Drawing for the job (mm, zero at the part's lowest x, y, z). A direction names the side the tool comes from. Round coordinates to 2 decimals unless told otherwise and drop trailing zeros. Write each loop counter-clockwise with the first axis right and the second up, starting at its lowest first coordinate (ties: lowest second). Pieces come first, ordered by that corner, then holes. Notation, with made-up numbers: (-34.5, 55.25) - (-2.5, 55.25) arc R29 ccw to (-2.5, 82.25) - close; hole circle Ø4 at (13.25, 15.5). An arc over 180 degrees is marked (long way). One line per question, with ' | ' between items.
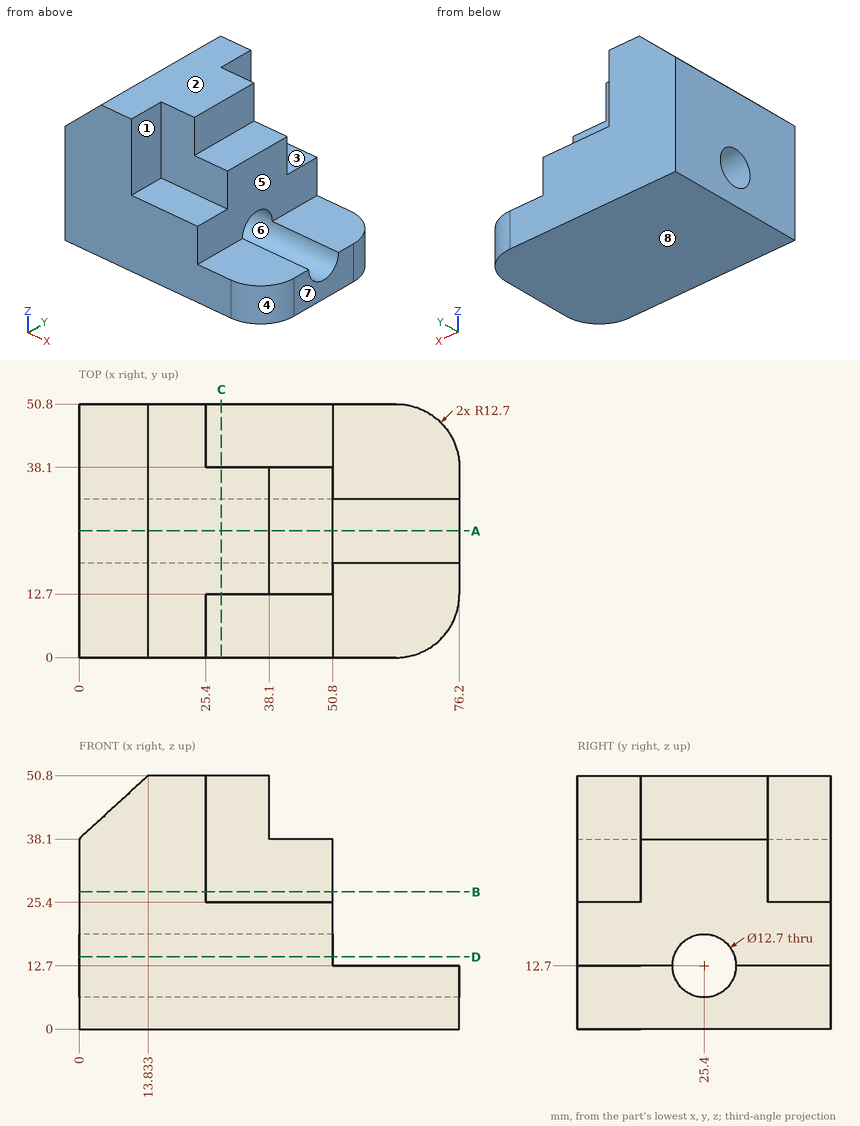
Q1. Drop flat-ended pins along their axis: pin 1 (10 mm diameter, centred on x = 39.5, y = 47.5, fed in from +Z); pin 2 (6.5 mm diameter, centred on y = 21.5, z = 46, fed in from +X); pin 3 (8 mm diameter, centred on y = 25.5, z = 10, fed in from +X); pin 4 (7.5 mm diameter, centred on y = 17.5, z = 27.5, fed in from +X). Give the stop position or say it passes through.
Found:
pin 1: z = 25.4 | pin 2: x = 38.1 | pin 3: x = 76.2 | pin 4: x = 50.8
Q2. Saw through at D-D, the plane z = 14.5. List the corners of the cut face in (x, y), then the cut area to 3 significant figures.
Found:
outline: (0, 0) - (50.8, 0) - (50.8, 19.31) - (0, 19.31) - close; (0, 31.49) - (50.8, 31.49) - (50.8, 50.8) - (0, 50.8) - close | area: 1,960 mm^2
Q3. Saw through at A-A, the plane y = 25.4. List the corners of the cut face in (x, z), then the cut area to 3 significant figures.
Found:
outline: (0, 0) - (76.2, 0) - (76.2, 6.35) - (0, 6.35) - close; (0, 19.05) - (50.8, 19.05) - (50.8, 38.1) - (38.1, 38.1) - (38.1, 50.8) - (13.83, 50.8) - (0, 38.1) - close | area: 1,850 mm^2
Q4. Saw through at B-B, the plane z = 27.5. List the corners of the cut face in (x, y), then the cut area to 3 significant figures.
Found:
outline: (0, 0) - (25.4, 0) - (25.4, 12.7) - (50.8, 12.7) - (50.8, 38.1) - (25.4, 38.1) - (25.4, 50.8) - (0, 50.8) - close | area: 1,940 mm^2
Q5. Saw through at C-C, the plane x = 28.5. List the corners of the cut face in (y, z).
Found:
outline: (0, 0) - (50.8, 0) - (50.8, 25.4) - (38.1, 25.4) - (38.1, 50.8) - (12.7, 50.8) - (12.7, 25.4) - (0, 25.4) - close; hole circle Ø12.7 at (25.4, 12.7)
Q6. Drill centre lines: L1, parallel to Z at x = 48.5, y = 25.4; L2, parallel to Y at x = 33, z = 12.7; L3, parallel to Z at x = 31, y = 25.4. Where is each one in solid material? Low to high. Write a range as from..to.
Found:
L1: 0..6.35, 19.05..38.1 | L2: 0..19.05, 31.75..50.8 | L3: 0..6.35, 19.05..50.8
Q7. Pull direction Z, two halves, no side cores. Call the marked faces 6, 7 and 8: +Z half, -Z half, draft (parallel to the pull), parting line (faces both ways), or undercut.
Found:
face 6: undercut | face 7: draft | face 8: -Z half
Q8. Which spindle directions (+Z, -Z, +X, -X, +Y, -Y) get a long thin tool onto all of the face, cutting with end or side? Do the marked faces 1, 2, 3, 4 and 5. Say none if no direction does.
Found:
face 1: +Z, +X, -Y | face 2: +Z, +X, -X, +Y, -Y | face 3: +Z, +X, +Y | face 4: +Z, -Z, +X, -Y | face 5: +Z, +X, +Y, -Y
